Check sheet for the modelled part. Datum: model origin and axes. Units: mm. A direction names the side the tool comes from. Round coordinates to 2 decimals unless told otherwise and drop trailing zeros. Order: outer loops, then holes, each group sorted by start corner. A loop starts at its lowest first (then second) coordinate and runs counter-clockwise, first axis right, second up.
from build123d import *

# Parameters (mm, degrees)
SKETCH1_W             = 76.2
SKETCH1_H             = 203.2
BOSS_EXTRUDE1_DEPTH   = 6.35
BOSS_EXTRUDE1_2_DEPTH = 6.35
SKETCH2_W             = 38.1
SKETCH2_H             = 76.2
BOSS_EXTRUDE2_DEPTH   = 889
SKETCH3_W             = 177.8
SKETCH3_H             = 38.1
BOSS_EXTRUDE3_DEPTH   = 76.2
BOSS_EXTRUDE4_REACH   = 777.766
SKETCH7_R             = 4
BOSS_EXTRUDE5_DEPTH   = 50


with BuildPart() as part:
    # Sketch1 → Boss-Extrude1 (new body)
    with BuildSketch(Plane(origin=(0, 0, 0), x_dir=(1, 0, 0), z_dir=(0, 1, 0))):
        with Locations((127, -101.6)):
            Rectangle(SKETCH1_W, SKETCH1_H)
    extrude(amount=BOSS_EXTRUDE1_DEPTH)



with BuildPart() as body_2:
    # Sketch1 → Boss-Extrude1 2 (new body)
    with BuildSketch(Plane(origin=(0, 0, 0), x_dir=(1, 0, 0), z_dir=(0, 1, 0))):
        with Locations((-127, -101.6)):
            Rectangle(SKETCH1_W, SKETCH1_H)
    extrude(amount=BOSS_EXTRUDE1_2_DEPTH)


with BuildPart() as part_1:
    add(part.part)

    add(body_2.part)  # Boss-Extrude2 merges body 2
    # Sketch2 → Boss-Extrude2 (add)
    with BuildSketch(Plane(origin=(0, 6.35, 0), x_dir=(1, 0, 0), z_dir=(0, 1, 0))):
        with Locations((-107.95, -101.6)):
            Rectangle(SKETCH2_W, SKETCH2_H)
        with Locations((107.95, -101.6)):
            Rectangle(SKETCH2_W, SKETCH2_H)
    extrude(amount=BOSS_EXTRUDE2_DEPTH)

    # Sketch3 → Boss-Extrude3 (add)
    with BuildSketch(Plane.XY.offset(139.7)):
        with Locations((0, 876.3)):
            Rectangle(SKETCH3_W, SKETCH3_H)
        with Locations((0, 711.2)):
            Rectangle(SKETCH3_W, SKETCH3_H)
    extrude(amount=-BOSS_EXTRUDE3_DEPTH)

    # Sketch6 → Boss-Extrude4 (add, up to next)
    with BuildSketch(Plane(origin=(0, 730.25, 0), x_dir=(1, 0, 0), z_dir=(0, 1, 0)), mode=Mode.PRIVATE) as boss_extrude4_sk1:
        Polygon((-3.75, -130.2), (-20.204482672, -139.7), (-20.829482672, -138.617468245), (-4.375, -129.117468245), align=None)
    boss_extrude4_tool1 = extrude(boss_extrude4_sk1.sketch, amount=BOSS_EXTRUDE4_REACH, mode=Mode.PRIVATE) - part_1.part
    # Sketch6 → Boss-Extrude4 (add, up to next)
    with BuildSketch(Plane(origin=(0, 730.25, 0), x_dir=(1, 0, 0), z_dir=(0, 1, 0)), mode=Mode.PRIVATE) as boss_extrude4_sk2:
        Polygon((20.829482672, -138.617468245), (20.204482672, -139.7), (3.75, -130.2), (4.375, -129.117468245), align=None)
    boss_extrude4_tool2 = extrude(boss_extrude4_sk2.sketch, amount=BOSS_EXTRUDE4_REACH, mode=Mode.PRIVATE) - part_1.part
    add(boss_extrude4_tool1.solids().sort_by_distance((-12.289741, 730.25, 134.408734))[0])
    add(boss_extrude4_tool2.solids().sort_by_distance((12.289741, 730.25, 134.408734))[0])

    # Sketch7 → Boss-Extrude5 (add)
    with BuildSketch(Plane(origin=(0, 730.25, 0), x_dir=(1, 0, 0), z_dir=(0, 1, 0))):
        with Locations(Location((15, -99.7, 0), (0, 0, 270))):
            Circle(SKETCH7_R)
    extrude(amount=BOSS_EXTRUDE5_DEPTH)


solid = part_1.part
1) Gauge pin test, flat ends, axial feed: pin 1 (23 mm diameter, centred on x = 144, z = 118, fed in from +Y); pin 2 (1 mm diameter, centred on x = -101.5, y = 251, fed in from -Z); pin 3 (10 mm diameter, centred on x = -126, y = 359.5, fed in from +Z). Record the tip position at first contact, or that the pin passes through.
2) Draft check along X on faces 6 (the face through (126, 0, 100)), 7 (the face through (-88.9, 793, 102)), 8 (the face through (127, 445, 102)). Enter one of: pulls with the +X half, pulls with the -X half, needs draft (parallel to the pull), parting line crosses it, or undercut.
3) Sectioned sample at D-D on x = -108. Record the cut outline in (y, z), and give its area (3 significant figures).
4) Sectioned sample at A-A on z = 166.5. Record the cut outline in (x, y), and give its area (3 significant figures).
5) Sectioned sample at B-B on y = 341.5. Record the cut outline in (x, z), and give its area (3 significant figures).
6) Set-up check for faces 1 (the face through (-95, 519, 139.7)), 2 (the face through (-95, 519, 63.5)), 3 (the face through (-11.862, 792.861, 134.884)), 4 (the face through (88.9, 793, 102)), 5 (the face through (88.9, 344, 95)): record each of +Z, -Z, +X, -X, +Y, -Y from which the full face is reachable in a straight line by a thin tool's end or side.
7) Scan lines: line 1 (Y direction, x = -20.5, z = 117); line 2 (Z direction, x = 126, y = 226.5); line 3 (Y direction, x = 97, z = 190.5). Record each from-to range of solid material in increasing order.
8) Sectioned sample at C-C on z = 73.5. Record the cut outline in (x, y).
Values found:
1. pin 1: stops at y = 6.35
1. pin 2: stops at z = 63.5
1. pin 3: stops at z = 139.7
2. face 6: needs draft
2. face 7: undercut
2. face 8: pulls with the +X half
3. outline: (0, 0) - (6.35, 0) - (6.35, 63.5) - (895.35, 63.5) - (895.35, 139.7) - (6.35, 139.7) - (6.35, 203.2) - (0, 203.2) - close
3. area: 69,000 mm2
4. outline: (-165.1, 0) - (-88.9, 0) - (-88.9, 6.35) - (-165.1, 6.35) - close; (88.9, 0) - (165.1, 0) - (165.1, 6.35) - (88.9, 6.35) - close
4. area: 968 mm2
5. outline: (-127, 63.5) - (-88.9, 63.5) - (-88.9, 139.7) - (-127, 139.7) - close; (88.9, 63.5) - (127, 63.5) - (127, 139.7) - (88.9, 139.7) - close
5. area: 5,810 mm2
6. face 1: +Z, +X, -X, +Y
6. face 2: -Z, +X, -X, +Y
6. face 3: +Z
6. face 4: +Z, -Z
6. face 5: +Z, -Z, -Y
7. line 1: y = 692.15 to 730.25, 857.25 to 895.35
7. line 2: z = 63.5 to 139.7
7. line 3: y = 0 to 6.35
8. outline: (-165.1, 0) - (-88.9, 0) - (-88.9, 692.15) - (88.9, 692.15) - (88.9, 0) - (165.1, 0) - (165.1, 6.35) - (127, 6.35) - (127, 895.35) - (-127, 895.35) - (-127, 6.35) - (-165.1, 6.35) - close; hole (-88.9, 730.25) - (88.9, 730.25) - (88.9, 857.25) - (-88.9, 857.25) - close
